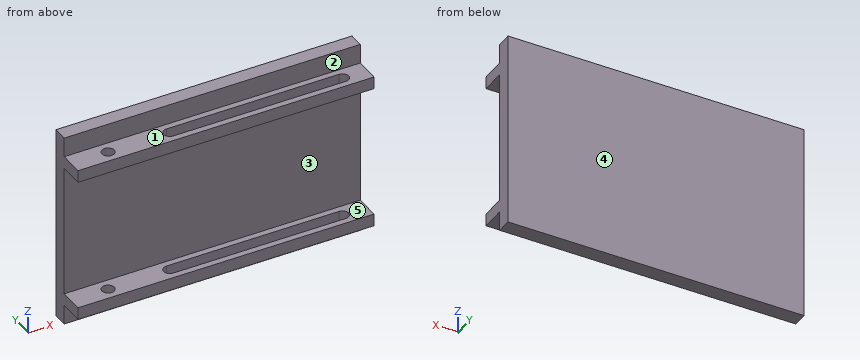
```python
from build123d import *

# Parameters (mm, degrees)
SKETCH_1_W          = 120
SKETCH_1_H          = 80
EXTRUDE_1_DEPTH     = 6
SKETCH_10_W         = 120
SKETCH_10_H         = 5
EXTRUDE_3_DEPTH     = 10
SKETCH_11_R         = 2.5
CUT_EXTRUDE_1_DEPTH = 5


with BuildPart() as part:
    # 草圖1 → 填料-伸長1 (new body)
    with BuildSketch(Plane(origin=(0, 0, 0), x_dir=(1, 0, 0), z_dir=(0, 1, 0))):
        Rectangle(SKETCH_1_W, SKETCH_1_H)
    extrude(amount=EXTRUDE_1_DEPTH)

    # 草圖10 → 填料-伸長3 (add)
    with BuildSketch(Plane.XZ):
        with Locations((0, 29.5)):
            Rectangle(SKETCH_10_W, SKETCH_10_H)
    extrude_3 = extrude(amount=EXTRUDE_3_DEPTH)

    # 草圖11 → 除料-伸長1 (cut)
    with BuildSketch(Plane.XY.offset(32)):
        with Locations((-45, -5)):
            Circle(SKETCH_11_R)
        with BuildLine():
            Line((-20, -2.5), (50, -2.5))
            ThreePointArc((50, -2.5), (52.5, -5), (50, -7.5))
            Line((50, -7.5), (-20, -7.5))
            ThreePointArc((-20, -7.5), (-22.5, -5), (-20, -2.5))
        make_face()
    cut_extrude_1 = extrude(amount=-CUT_EXTRUDE_1_DEPTH, mode=Mode.SUBTRACT)

    # 鏡射3: 填料-伸長3, 除料-伸長1 across plane
    add(extrude_3.mirror(Plane.XY))
    add(cut_extrude_1.mirror(Plane.XY), mode=Mode.SUBTRACT)


solid = part.part
```
Here's how the part is built. I have some questions about the finished solid (model axes, mm). Face numbers are marked on the shaded views. A direction names the side the tool comes from. Coordinates: 2 decimals unless noted, no trailing zeros. Order: outer loops, then holes, each group sorted by start corner. A loop starts at its lowest first (then second) coordinate and runs counter-clockwise, first axis right, second up.
Item 1: I'm going to push flat-ended pins straight in: pin 1 Ø6.5 at (x, y) = (-45, -5) entering from +Z; pin 2 Ø9 at (x, z) = (9.5, 35.5) entering from -Y; pin 3 Ø3 at (x, y) = (-3, -6.5) entering from -Z; pin 4 Ø2.5 at (x, z) = (17.5, -37.5) entering from -Y. Where does each tip first touch, or does it pass through?
Response values:
pin 1: stops at z = 32
pin 2: stops at y = -10
pin 3: stops at z = -32
pin 4: stops at y = 0
Item 2: Thinking about a two-plate mould opening in Z: for the marked faces 1, 2 and 3, which applies, pulls with the +Z half, pulls with the -Z half, needs draft (parallel to the pull), parting line crosses it, or undercut?
Response values:
face 1: pulls with the +Z half
face 2: needs draft
face 3: undercut
Item 3: If we section it at A-A, the plane y = -5: List the corners of the cut face in (x, z) for me.
Response values:
outline: (-60, -32) - (-47.5, -32) - (-47.5, -27) - (-60, -27) - close; (-60, 27) - (-47.5, 27) - (-47.5, 32) - (-60, 32) - close; (-42.5, -32) - (-22.5, -32) - (-22.5, -27) - (-42.5, -27) - close; (-42.5, 27) - (-22.5, 27) - (-22.5, 32) - (-42.5, 32) - close; (52.5, -32) - (60, -32) - (60, -27) - (52.5, -27) - close; (52.5, 27) - (60, 27) - (60, 32) - (52.5, 32) - close
Item 4: Which directions (+Z, -Z, +X, -X, +Y, -Y) give clear straight access to the entire face, cutting with the end or side of a thin tool? Please do the marked faces 4 and 5.
Response values:
face 4: +Z, -Z, +X, -X, +Y
face 5: +X, -X, -Y
Item 5: I need wall thicknesses on probe 1 along Y at (x, z) = (-45, 30.1); probe 2 along Z at (x, y) = (33.5, -1); probe 3 along Y at (x, z) = (17.5, 20). Which ranges of each line are inside material? Lowest first, please.
Response values:
probe 1: y = -10 to -7.5, -2.5 to 6
probe 2: z = -32 to -27, 27 to 32
probe 3: y = 0 to 6
Item 6: If we section it at C-C, the plane z = 15: List the corners of the cut face in (x, y) for me.
Response values:
outline: (-60, 0) - (60, 0) - (60, 6) - (-60, 6) - close
Item 7: If we section it at B-B, the plane x = -45: List the corners of the cut face in (y, z) for me, then the cut area to 3 significant figures.
Response values:
outline: (-10, -32) - (-7.5, -32) - (-7.5, -27) - (-10, -27) - close; (-10, 27) - (-7.5, 27) - (-7.5, 32) - (-10, 32) - close; (-2.5, -32) - (0, -32) - (0, -40) - (6, -40) - (6, 40) - (0, 40) - (0, 32) - (-2.5, 32) - (-2.5, 27) - (0, 27) - (0, -27) - (-2.5, -27) - close
area: 530 mm2
